```python
from build123d import *

# Parameters (mm, degrees)
SKETCH1_W           = 60.5
SKETCH1_H           = 37
BOSS_EXTRUDE1_DEPTH = 2
SKETCH2_W           = 57.01
SKETCH2_H           = 29.41
CUT_EXTRUDE1_DEPTH  = 0.1
FILLET1_R           = 0.5
FILLET2_R           = 0.2
FILLET3_R           = 0.05


with BuildPart() as part:
    # Sketch1 → Boss-Extrude1 (new body)
    with BuildSketch(Plane(origin=(0, 0, 0), x_dir=(1, 0, 0), z_dir=(0, 1, 0))):
        with Locations((30.25, 18.5)):
            Rectangle(SKETCH1_W, SKETCH1_H)
    extrude(amount=BOSS_EXTRUDE1_DEPTH)

    # Sketch2 → Cut-Extrude1 (cut)
    with BuildSketch(Plane(origin=(0, 2, 0), x_dir=(1, 0, 0), z_dir=(0, 1, 0))):
        with Locations((30.25, 20.495)):
            Rectangle(SKETCH2_W, SKETCH2_H)
    extrude(amount=-CUT_EXTRUDE1_DEPTH, mode=Mode.SUBTRACT)

    # Fillet1
    fillet1_edges = [part.edges().sort_by_distance(p)[0] for p in [
        (0, 1, 0),
        (60.5, 1, 0),
        (60.5, 1, -37),
        (0, 1, -37),
    ]]
    fillet(fillet1_edges, radius=FILLET1_R)

    # Fillet2
    fillet2_edges = [part.edges().sort_by_distance(p)[0] for p in [
        (30.25, 2, 0),
        (0, 2, -18.5),
        (60.5, 2, -18.5),
        (30.25, 2, -37),
        (0.146446609, 2, -36.853553391),
        (60.353553391, 2, -36.853553391),
        (60.353553391, 2, -0.146446609),
        (0.146446609, 2, -0.146446609),
    ]]
    fillet(fillet2_edges, radius=FILLET2_R)

    # Fillet3
    fillet3_edges = [part.edges().sort_by_distance(p)[0] for p in [
        (1.745, 2, -20.495),
        (30.25, 2, -5.79),
        (58.755, 2, -20.495),
        (30.25, 2, -35.2),
    ]]
    fillet(fillet3_edges, radius=FILLET3_R)


solid = part.part
```
Geometry: final body of the model. Coordinates: model frame, mm. Round coordinates to 2 decimals unless told otherwise and drop trailing zeros. Order: outer loops, then holes, each group sorted by start corner. A loop starts at its lowest first (then second) coordinate and runs counter-clockwise, first axis right, second up. Notation, with made-up numbers: (52.5, 67) -> (67.5, 67) arc R19 ccw to (67.5, 103) -> close; hole circle Ø4 at (-23.5, 85). An arc over 180 degrees is marked (long way). Use one line per item in the form item = value. Start each with the question number.
1. Cut plane A-A (x = 49.5). Return the cut outline in (y, z).
2. Pin query (flat end, axial travel): pin 1 Ø14.5 at (x, z) = (17, -27) entering from +Y. Return the tip coordinate at first contact, or that it passes through.
3. Draft query along Z for faces 1 (the face through (30, 1, 0)), 2 (the face through (30, 1.9, -21)), 3 (the face through (0, 1, -18)). Return one class per face: pulls with the +Z half, pulls with the -Z half, needs draft (parallel to the pull), parting line crosses it, or undercut.
4. Cut plane B-B (z = -33). Return the cut outline in (x, y) (3 decimals), then the cut area to 3 significant figures.
5. Line query: probe 1 along Y at (x, z) = (29.5, -16.5). Output: solid intervals per line, ascending.
Solution:
q1.outline = (0, -37) -> (1.8, -37) arc R0.2 ccw to (2, -36.8) -> (2, -35.25) arc R0.05 ccw to (1.95, -35.2) -> (1.9, -35.2) -> (1.9, -5.79) -> (1.95, -5.79) arc R0.05 ccw to (2, -5.74) -> (2, -0.2) arc R0.2 ccw to (1.8, 0) -> (0, 0) -> close
q2.pin_1 = 1.9
q3.face_1 = pulls with the +Z half
q3.face_2 = undercut
q3.face_3 = needs draft
q4.outline = (0, 0) -> (60.5, 0) -> (60.5, 1.8) arc R0.2 ccw to (60.3, 2) -> (58.805, 2) arc R0.05 ccw to (58.755, 1.95) -> (58.755, 1.9) -> (1.745, 1.9) -> (1.745, 1.95) arc R0.05 ccw to (1.695, 2) -> (0.2, 2) arc R0.2 ccw to (0, 1.8) -> close
q4.area = 115 mm^2
q5.probe_1 = 0 to 1.9
